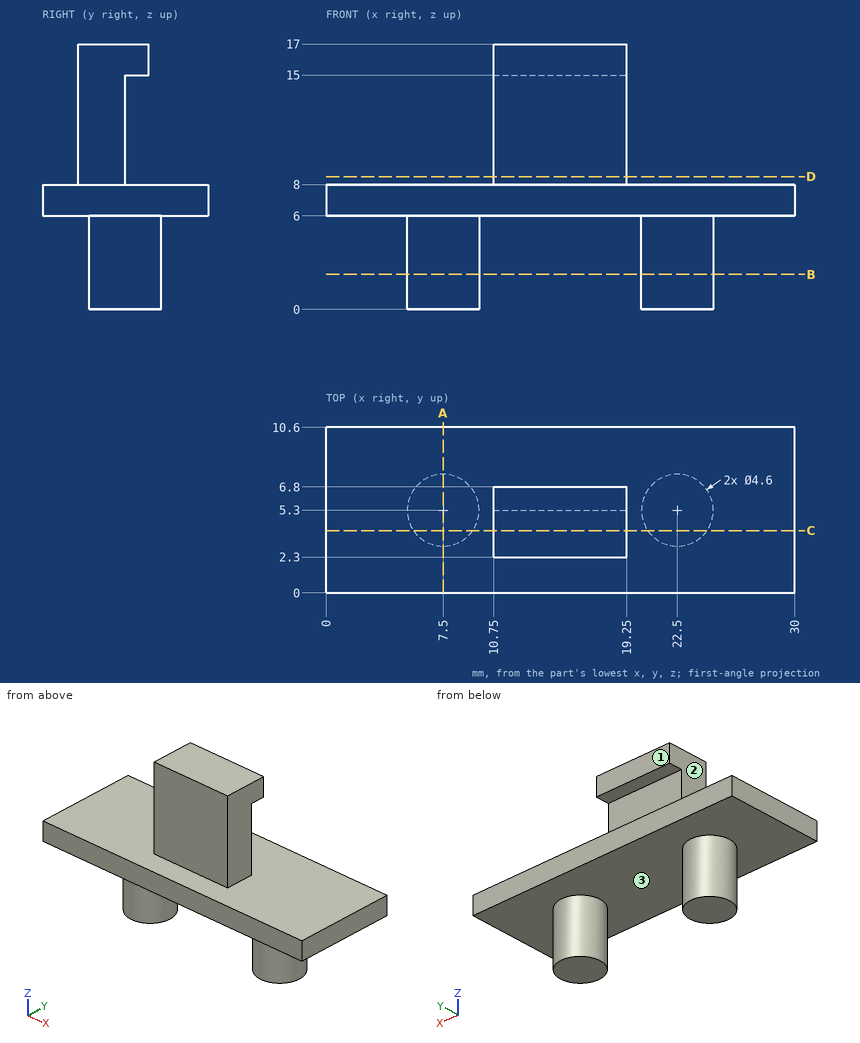
Check sheet for the drawn part. Datum: minimum x, y, z corner. Units: mm. A direction names the side the tool comes from. Coordinates: 2 decimals unless noted, no trailing zeros. Order: outer loops, then holes, each group sorted by start corner. A loop starts at its lowest first (then second) coordinate and runs counter-clockwise, first axis right, second up. Notation, with made-up numbers: M -3.5,8 L 47.5,8 A19 ccw 47.5,27 Z; hole C 37,49.5 d11. An arc over 180 degrees is marked long. One line per item, written item: value. Start each with the question number.
Item 1: Sectioned sample at A-A (x = 7.5). Enter the section's corners in (y, z).
Item 2: Scan lines: probe 1 along Z at (x, y) = (15, 6.5); probe 2 along X at (y, z) = (4.5, 5.75); probe 3 along Z at (x, y) = (25, 7.25). Record each from-to range of solid material in increasing order.
Item 3: Access from +Z, -Z, +X, -X, +Y, -Y to the whole of each face (thin tool, end or side, straight path). Record for the marked faces 1, 2 and 3.
Item 4: Sectioned sample at C-C (y = 4). Enter the section's corners in (x, z), then the cut area to 3 significant figures.
Item 5: Gauge pin test, flat ends, axial feed: pin 1 (3.5 mm diameter, centred on y = 3.5, z = 14, fed in from +X); pin 2 (7 mm diameter, centred on x = 16.5, z = 13.5, fed in from -Y); pin 3 (3.5 mm diameter, centred on x = 14, z = 13, fed in from +Y); pin 4 (3 mm diameter, centred on x = 17, y = 8, fed in from +Z). Record the tip position at first contact, or that the pin passes through.
Item 6: Sectioned sample at D-D (z = 8.5). Enter the section's corners in (x, y).
Item 7: Sectioned sample at B-B (z = 2.25). Enter the section's corners in (x, y), then the cut area to 3 significant figures.
Conclusion:
1. outline: M 0,6 L 3,6 L 3,0 L 7.6,0 L 7.6,6 L 10.6,6 L 10.6,8 L 0,8 Z
2. probe 1: z = 6 to 8, 15 to 17
2. probe 2: x = 5.34 to 9.66, 20.34 to 24.66
2. probe 3: z = 6 to 8
3. face 1: +Z, +X, -X, +Y
3. face 2: +Z, -X, +Y, -Y
3. face 3: -Z
4. outline: M 0,6 L 5.6,6 L 5.6,0 L 9.4,0 L 9.4,6 L 20.6,6 L 20.6,0 L 24.4,0 L 24.4,6 L 30,6 L 30,8 L 19.25,8 L 19.25,17 L 10.75,17 L 10.75,8 L 0,8 Z
4. area: 182 mm^2
5. pin 1: stops at x = 19.25
5. pin 2: stops at y = 2.3
5. pin 3: stops at y = 5.3
5. pin 4: stops at z = 17
6. outline: M 10.75,2.3 L 19.25,2.3 L 19.25,5.3 L 10.75,5.3 Z
7. outline: C 7.5,5.3 d4.6; C 22.5,5.3 d4.6
7. area: 33.2 mm^2
